from build123d import *

# Parameters (mm, degrees)
SKETCH001_W  = 0.48
SKETCH001_H  = 0.38
PAD001_DEPTH = 5
PAD_DEPTH    = 4.8


with BuildPart() as pad001:
    # Sketch001 → Pad001 (new body)
    with BuildSketch(Plane.XY.offset(2.5)):
        Rectangle(SKETCH001_W, SKETCH001_H)
        with Locations((1.27, 0)):
            Rectangle(SKETCH001_W, SKETCH001_H)
        with Locations((2.54, 0)):
            Rectangle(SKETCH001_W, SKETCH001_H)
    extrude(amount=-PAD001_DEPTH)


with BuildPart() as to_92_inline_narrow:
    # Sketch → Pad (new body)
    with BuildSketch(Plane.XY.offset(2.5)):
        with BuildLine():
            Line((-0.745769, -1.33), (3.285769, -1.33))
            ThreePointArc((3.285769, -1.33), (1.27, 2.415), (-0.745769, -1.33))
        make_face()
    extrude(amount=PAD_DEPTH)

    add(pad001.part)


solid = to_92_inline_narrow.part
Could you check a few things on this model? Use its own coordinates, in mm. Coordinates: 2 decimals unless noted, no trailing zeros. Loops run counter-clockwise (first coordinate to the right, second up) from the corner with the lowest first, then second, coordinate; pieces in that order, holes last. Notation, with made-up numbers: (-22.75, 15) -> (-12.75, 15) arc R15 cw to (-12.75, 31) -> close; hole circle Ø1 at (43.5, 83.25). An arc over 180 degrees is marked (long way). Answer in a Markdown table with one row per item.
(1) Will these pins go through, and if not, where does the flat tip stop? pin 1 Ø2 at (x, y) = (0.5, -0.5) entering from -Z; pin 2 Ø1 at (y, z) = (2, 6) entering from -X; pin 3 Ø0.5 at (x, z) = (1.5, -0.5) entering from +Y.
Results found:
| item | result |
|---|---|
| pin 1 | stops at z = -2.5 |
| pin 2 | stops at x = -0.62 |
| pin 3 | stops at y = 0.19 |
(2) If I drill on probe 1 along X at (y, z) = (0, 1.75); probe 2 along Z at (x, y) = (0.75, -0.6); probe 3 along Y at (x, z) = (2.6, -1.5), over which ranges is the centre line in solid material (lowest first)?
Results found:
| item | result |
|---|---|
| probe 1 | x = -0.24 to 0.24, 1.03 to 1.51, 2.3 to 2.78 |
| probe 2 | z = 2.5 to 7.3 |
| probe 3 | y = -0.19 to 0.19 |
(3) Imagine slicing it at A-A (z = -1.25). List the corners of the cut face in (x, y) for me, plus the area to 3 significant figures.
Results found:
| item | result |
|---|---|
| outline | (-0.24, -0.19) -> (0.24, -0.19) -> (0.24, 0.19) -> (-0.24, 0.19) -> close; (1.03, -0.19) -> (1.51, -0.19) -> (1.51, 0.19) -> (1.03, 0.19) -> close; (2.3, -0.19) -> (2.78, -0.19) -> (2.78, 0.19) -> (2.3, 0.19) -> close |
| area | 0.547 mm^2 |
(4) Imagine slicing it at C-C (y = 0). List the corners of the cut face in (x, z) for me (3 decimals).
Results found:
| item | result |
|---|---|
| outline | (-1.145, 2.5) -> (-0.24, 2.5) -> (-0.24, -2.5) -> (0.24, -2.5) -> (0.24, 2.5) -> (1.03, 2.5) -> (1.03, -2.5) -> (1.51, -2.5) -> (1.51, 2.5) -> (2.3, 2.5) -> (2.3, -2.5) -> (2.78, -2.5) -> (2.78, 2.5) -> (3.685, 2.5) -> (3.685, 7.3) -> (-1.145, 7.3) -> close |
(5) Imagine slicing it at B-B (x = 1.27). List the corners of the cut face in (y, z) for me (3 decimals), plus the area to 3 significant figures.
Results found:
| item | result |
|---|---|
| outline | (-1.33, 2.5) -> (-0.19, 2.5) -> (-0.19, -2.5) -> (0.19, -2.5) -> (0.19, 2.5) -> (2.415, 2.5) -> (2.415, 7.3) -> (-1.33, 7.3) -> close |
| area | 19.9 mm^2 |
(6) Imagine slicing it at D-D (z = 6.75). List the corners of the cut face in (x, y) for me (3 decimals).
Results found:
| item | result |
|---|---|
| outline | (-0.746, -1.33) -> (3.286, -1.33) arc R2.415 ccw (long way) to start |
